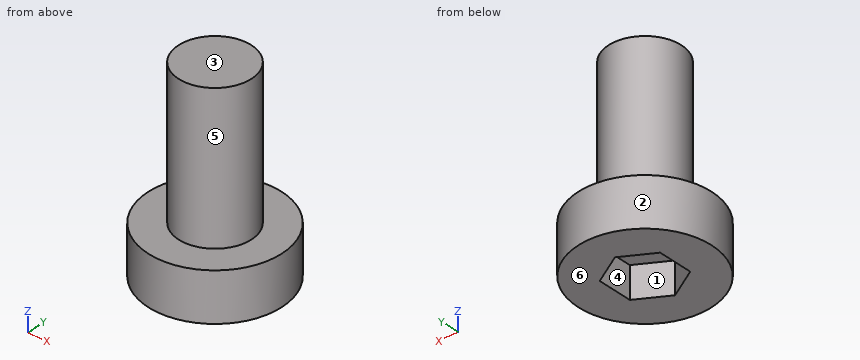
Autodesk Inventor part; units mm, degrees
ref_plane "YZ Plane" through (0, 0, 0) normal (1, 0, 0) x (0, 1, 0)
ref_plane "XZ Plane" through (0, 0, 0) normal (0, 1, 0) x (-1, 0, 0)
ref_plane "XY Plane" through (0, 0, 0) normal (0, 0, 1) x (1, 0, 0)
sketch "スケッチ1" plane through (0, 0, 0) normal (1, 0, 0) x (0, 1, 0)
  line L0 (0, 8) -> (0, 0)
  line L1 (0, 0) -> (2.75, 0)
  line L2 (2.75, 0) -> (2.75, 2)
  line L3 (2.75, 2) -> (1.5, 2)
  line L4 (1.5, 2) -> (1.5, 8)
  line L5 (1.5, 8) -> (0, 8)
  dimension "d2" = 2
  dimension "d10" = 6
  dimension "d11" = 3
  dimension "d12" = 5.5
revolve "回転1" add sketch "スケッチ1" angle 360 about axis through (0, 0, 8) along (0, 0, -1)
thread "ねじ1"
sketch "スケッチ2" plane through (0, 0, 0) normal (0, 0, -1) x (-1, 0, 0)
  line L0 (0, 1.4434) -> (1.25, 0.7217)
  line L1 (1.25, 0.7217) -> (1.25, -0.7217)
  line L2 (1.25, -0.7217) -> (0, -1.4434)
  line L3 (0, -1.4434) -> (-1.25, -0.7217)
  line L4 (-1.25, -0.7217) -> (-1.25, 0.7217)
  line L5 (-1.25, 0.7217) -> (0, 1.4434)
  circle A0 centre (0, 0) radius 2.75
  line L6 (0, 2.75) -> (0, -2.75) construction
  point P0 (0, 0)
  dimension "d7" = 2.5
extrude "押し出し1" cut sketch "スケッチ2" against normal blind 1.3 contours L0 L1 L2 L3 L4 L5
properties part number "LowHead_M3-6" material "ステンレス鋼 AISI 304"
Input: part model. Units: mm. Frame: model coordinates. Face numbers are marked on the shaded views. A direction names the side the tool comes from. Give positions to 0.01 mm unless a question says otherwise; leave off trailing zeros. Loops run counter-clockwise (first coordinate to the right, second up) from the corner with the lowest first, then second, coordinate; pieces in that order, holes last.
1) Line query: L1, parallel to X at y = 0.65, z = 0.5; L2, parallel to Z at x = -2.1, y = -0.7; L3, parallel to Y at x = 0.05, z = 2.25. Output: solid intervals per line, ascending.
A:
L1: x = -2.67 to -1.25, 1.25 to 2.67
L2: z = 0 to 2
L3: y = -1.5 to 1.5
2) Contact query for flat-ended pins moving along their axis: pin 1 (3 mm diameter, centred on x = 0, z = 5, fed in from -Y); pin 2 (1.3 mm diameter, centred on x = 0, y = 0, fed in from -Z); pin 3 (3 mm diameter, centred on x = 1.5, z = 6, fed in from +Y). Output: stop coordinate, or through.
A:
pin 1: stops at y = -1.5
pin 2: stops at z = 1.3
pin 3: stops at y = 1.5
3) Section query C-C on x = -0.6. Return the cut outline in (y, z).
A:
outline: (-2.68, 0) - (-1.1, 0) - (-1.1, 1.3) - (1.1, 1.3) - (1.1, 0) - (2.68, 0) - (2.68, 2) - (1.37, 2) - (1.37, 8) - (-1.37, 8) - (-1.37, 2) - (-2.68, 2) - close
4) Section query D-D on z = 6.25. Return the cut outline in (x, y), and give its area (3 significant figures).
A:
outline: circle Ø3 at (0, 0)
area: 7.07 mm2
5) Mould query, pull axis Y, two halves, no side actions, for the marked faces 1, 2 and 3. Classes: released by +Y, released by -Y, zero draft, split by the parting line, or undercut.
A:
face 1: undercut
face 2: split by the parting line
face 3: zero draft
6) Section query A-A on z = 0.75. Return the cut outline in (x, y), and give its area (3 significant figures).
A:
outline: circle Ø5.5 at (0, 0); hole (-1.25, -0.72) - (0, -1.44) - (1.25, -0.72) - (1.25, 0.72) - (0, 1.44) - (-1.25, 0.72) - close
area: 18.3 mm2
7) Section query B-B on y = 0. Return the cut outline in (x, z), and give its area (4 significant figures).
A:
outline: (-2.75, 0) - (-1.25, 0) - (-1.25, 1.3) - (1.25, 1.3) - (1.25, 0) - (2.75, 0) - (2.75, 2) - (1.5, 2) - (1.5, 8) - (-1.5, 8) - (-1.5, 2) - (-2.75, 2) - close
area: 25.75 mm2
8) Reachability of the marked faces 4, 5 and 6 from +Z, -Z, +X, -X, +Y, -Y: full face, straight path, thin tool, end or side. Return the list, or none.
A:
face 4: -Z
face 5: +Z
face 6: -Z, +X, -X, +Y, -Y
